from build123d import *

# Parameters (mm, degrees)
SKETCH1_R           = 1.5
BOSS_EXTRUDE1_DEPTH = 15
BOSS_EXTRUDE2_DEPTH = 1.5


with BuildPart() as part:
    # Sketch1 → Boss-Extrude1 (new body)
    with BuildSketch(Plane(origin=(0, 0, 0), x_dir=(1, 0, 0), z_dir=(0, 1, 0))):
        Circle(SKETCH1_R)
    extrude(amount=BOSS_EXTRUDE1_DEPTH)

    # Sketch2 → Boss-Extrude2 (add)
    with BuildSketch(Plane.XZ):
        Polygon((2.5, 0.018896825), (1.23363487, 2.174511922), (-1.26636513, 2.155615097), (-2.5, -0.018896825), (-1.23363487, -2.174511922), (1.26636513, -2.155615097), align=None)
    extrude(amount=BOSS_EXTRUDE2_DEPTH)


solid = part.part
Source: CAD feature listing. Evaluate the final solid. Frame: model axes, mm. A direction names the side the tool comes from. Round coordinates to 2 decimals unless told otherwise and drop trailing zeros. Loops run counter-clockwise (first coordinate to the right, second up) from the corner with the lowest first, then second, coordinate; pieces in that order, holes last.
Q1. Ray query, line 1 (X direction, y = 4.25, z = 0); line 2 (X direction, y = 12, z = 0.8); line 3 (Y direction, x = 1.15, z = -1.2). Return the intervals inside material, ascending.
Q2. Section A-A, the plane z = -0.55. Return loops of the section in (x, y).
Q3. Access query for faces 1 (the face through (-1.5, 7.4, -0.07)), 2 (the face through (1.876, -0.74, 1.082)). Directions: +Z, -Z, +X, -X, +Y, -Y. A direction counts if a zero-diameter tool reaches every point of the face in a straight line with its end or side. Return the directions, or none.
Q4. Section B-B, the plane x = -0.8. Return loops of the section in (y, z).
Q5. Section D-D, the plane x = -1.7. Return loops of the section in (y, z), plus the area to 3 significant figures.
Q6. Section C-C, the plane y = 3.5. Return loops of the section in (x, z), plus the area to 3 significant figures.
Solutions:
1. line 1: x = -1.5 to 1.5
1. line 2: x = -1.27 to 1.27
1. line 3: y = -1.5 to 0
2. outline: (-2.19, -1.5) - (2.18, -1.5) - (2.18, 0) - (1.4, 0) - (1.4, 15) - (-1.4, 15) - (-1.4, 0) - (-2.19, 0) - close
3. face 1: +Y
3. face 2: +Z, +X, +Y, -Y
4. outline: (-1.5, -2.17) - (0, -2.17) - (0, -1.27) - (15, -1.27) - (15, 1.27) - (0, 1.27) - (0, 2.16) - (-1.5, 2.16) - close
5. outline: (-1.5, -1.38) - (0, -1.38) - (0, 1.39) - (-1.5, 1.39) - close
5. area: 4.16 mm2
6. outline: circle Ø3 at (0, 0)
6. area: 7.07 mm2
